Source: CAD feature listing. Evaluate the final solid. Frame: model axes, mm. Face numbers are marked on the shaded views. Round coordinates to 2 decimals unless told otherwise and drop trailing zeros. Write each loop counter-clockwise with the first axis right and the second up, starting at its lowest first coordinate (ties: lowest second). Pieces come first, ordered by that corner, then holes. Notation, with made-up numbers: (82, 28) -> (90, 28) arc R16 cw to (90, 39) -> close; hole circle Ø6 at (48, 84.25). An arc over 180 degrees is marked (long way). Put each result on its own line as item: value.
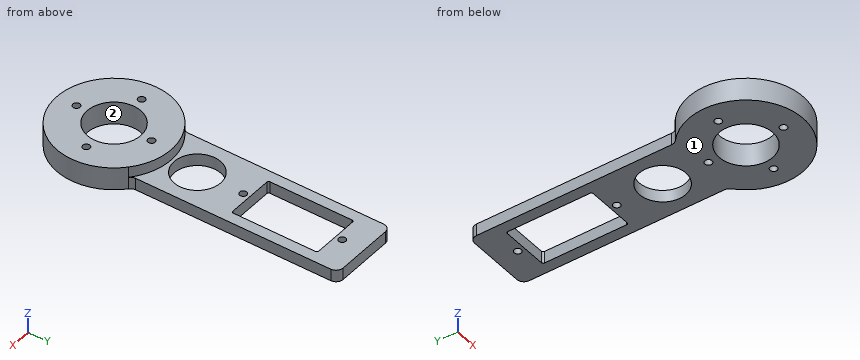
```python
from build123d import *
from build123d.topology import SkipClean

# Parameters (mm, degrees)
SKETCH1_R           = 1
BOSS_EXTRUDE1_DEPTH = 6.35
SKETCH2_R           = 1
SKETCH2_W           = 13.9
SKETCH2_H           = 24
CUT_EXTRUDE1_DEPTH  = 73.085522125
FILLET1_R           = 0.5
FILLET2_R           = 2
SKETCH3_R           = 6.5
CUT_EXTRUDE2_DEPTH  = 6.35
SKETCH4_R           = 7.5
CUT_EXTRUDE3_DEPTH  = 73.085522125
SKETCH5_R           = 6.5
SKETCH5_R_2         = 1
CUT_EXTRUDE4_DEPTH  = 3


with BuildPart() as part:
    # Sketch1 → Boss-Extrude1 (new body)
    with BuildSketch(Plane.XY):
        with BuildLine():
            Line((-10, 12.489995997), (-10, 70))
            Line((-10, 70), (10, 70))
            Line((10, 70), (10, 12.489995997))
            ThreePointArc((10, 12.489995997), (0, -16), (-10, 12.489995997))
        make_face()
        with Locations((-10.5, 0)):
            Circle(SKETCH1_R, mode=Mode.SUBTRACT)
        with Locations((0, 10.5)):
            Circle(SKETCH1_R, mode=Mode.SUBTRACT)
        with Locations((10.5, 0)):
            Circle(SKETCH1_R, mode=Mode.SUBTRACT)
        with Locations((0, -10.5)):
            Circle(SKETCH1_R, mode=Mode.SUBTRACT)
    extrude(amount=BOSS_EXTRUDE1_DEPTH)

    # Sketch2 → Cut-Extrude1 (cut, through all)
    with BuildSketch(Plane.XY.offset(6.35)):
        with Locations((0, 63.85)):
            Circle(SKETCH2_R)
        with Locations((0, 36.15)):
            Circle(SKETCH2_R)
        with Locations((0, 50)):
            Rectangle(SKETCH2_W, SKETCH2_H)
    extrude(amount=-CUT_EXTRUDE1_DEPTH, mode=Mode.SUBTRACT)

    # Fillet1
    fillet1_edges = [part.edges().sort_by_distance(p)[0] for p in [
        (6.95, 38, 3.175),
        (-6.95, 38, 3.175),
        (-6.95, 62, 3.175),
        (6.95, 62, 3.175),
    ]]
    fillet(fillet1_edges, radius=FILLET1_R)

    # Fillet2
    fillet2_edges = [part.edges().sort_by_distance(p)[0] for p in [
        (-10, 12.489995997, 3.175),
        (-10, 70, 3.175),
        (10, 70, 3.175),
        (10, 12.489995997, 3.175),
    ]]
    fillet(fillet2_edges, radius=FILLET2_R)

    # Sketch3 → Cut-Extrude2 (cut)
    with BuildSketch(Plane.XY.offset(6.35)):
        with Locations((0, 23.325)):
            Circle(SKETCH3_R)
    extrude(amount=-CUT_EXTRUDE2_DEPTH, mode=Mode.SUBTRACT)

    # Sketch4 → Cut-Extrude3 (cut, through all)
    with BuildSketch(Plane.XY.offset(6.35)):
        Circle(SKETCH4_R)
    extrude(amount=-CUT_EXTRUDE3_DEPTH, mode=Mode.SUBTRACT)

    # Sketch5 → Cut-Extrude4 (cut)
    with SkipClean():  # the faces are left unmerged after this step: merging them gives an invalid solid
        with BuildSketch(Plane.XY.offset(6.35)):
            with BuildLine():
                ThreePointArc((-10.666666667, 11.92569588), (0, 16), (10.666666667, 11.92569588))
                ThreePointArc((10.666666667, 11.92569588), (10.174258142, 12.599911284), (10, 13.416407865))
                Line((10, 13.416407865), (10, 68))
                ThreePointArc((10, 68), (9.414213562, 69.414213562), (8, 70))
                Line((8, 70), (-8, 70))
                ThreePointArc((-8, 70), (-9.414213562, 69.414213562), (-10, 68))
                Line((-10, 68), (-10, 13.416407865))
                ThreePointArc((-10, 13.416407865), (-10.174258142, 12.599911284), (-10.666666667, 11.92569588))
            make_face()
            with Locations((0, 23.325)):
                Circle(SKETCH5_R, mode=Mode.SUBTRACT)
            with Locations((0, 63.85)):
                Circle(SKETCH5_R_2, mode=Mode.SUBTRACT)
            with Locations((0, 36.15)):
                Circle(SKETCH5_R_2, mode=Mode.SUBTRACT)
            with BuildLine():
                ThreePointArc((6.45, 62), (6.803553391, 61.853553391), (6.95, 61.5))
                Line((6.95, 61.5), (6.95, 38.5))
                ThreePointArc((6.95, 38.5), (6.803553391, 38.146446609), (6.45, 38))
                Line((6.45, 38), (-6.45, 38))
                ThreePointArc((-6.45, 38), (-6.803553391, 38.146446609), (-6.95, 38.5))
                Line((-6.95, 38.5), (-6.95, 61.5))
                ThreePointArc((-6.95, 61.5), (-6.803553391, 61.853553391), (-6.45, 62))
                Line((-6.45, 62), (6.45, 62))
            make_face(mode=Mode.SUBTRACT)
        extrude(amount=-CUT_EXTRUDE4_DEPTH, mode=Mode.SUBTRACT)


solid = part.part
```
Q1. Cut plane A-A on x = 0. Give the number of separate pieces and of enclosed holes in the cut face, and give its area (3 significant figures).
Ans:
separate pieces: 8
enclosed holes: 0
area: 126 mm^2
Q2. Cut plane C-C on y = 0. Output: boundary loops of the cut face in (x, z), and give its area (4 significant figures).
Ans:
outline: (-16, 0) -> (-11.5, 0) -> (-11.5, 6.35) -> (-16, 6.35) -> close; (-9.5, 0) -> (-7.5, 0) -> (-7.5, 6.35) -> (-9.5, 6.35) -> close; (7.5, 0) -> (9.5, 0) -> (9.5, 6.35) -> (7.5, 6.35) -> close; (11.5, 0) -> (16, 0) -> (16, 6.35) -> (11.5, 6.35) -> close
area: 82.55 mm^2
Q3. Cut plane D-D on z = 5. Output: boundary loops of the cut face in (x, y), and give its area (3 significant figures).
Ans:
outline: circle Ø32 at (0, 0); hole circle Ø2 at (-10.5, 0); hole circle Ø15 at (0, 0); hole circle Ø2 at (0, -10.5); hole circle Ø2 at (0, 10.5); hole circle Ø2 at (10.5, 0)
area: 615 mm^2
Q4. Cut plane B-B on y = 36.15. Output: boundary loops of the cut face in (x, z).
Ans:
outline: (-10, 0) -> (-1, 0) -> (-1, 3.35) -> (-10, 3.35) -> close; (1, 0) -> (10, 0) -> (10, 3.35) -> (1, 3.35) -> close
Q5. Pin query (flat end, axial travel): pin 1 (1 mm diameter, centred on x = 7, y = 15.5, fed in from -Z); pin 2 (1.5 mm diameter, centred on x = 11.5, z = 3, fed in from +Y); pin 3 (6.5 mm diameter, centred on x = 0, y = 30, fed in from +Z); pin 4 (1.7 mm diameter, centred on y = 50.5, z = 2, fed in from -X). Return the tip coordinate at first contact, or that it passes through.
Ans:
pin 1: stops at z = 0
pin 2: stops at y = 11.85
pin 3: stops at z = 3.35
pin 4: stops at x = -10
Q6. Material intervals for line 1 (Y direction, x = -3, z = 3); line 2 (Y direction, x = 5.5, z = 3.25); line 3 (Y direction, x = 10.5, z = 4.5), sorted ascending. Write a range as [from, to].
Ans:
line 1: y = [-15.72, -6.87], [6.87, 17.56], [29.09, 38], [62, 70]
line 2: y = [-15.02, -5.1], [5.1, 19.86], [26.79, 38], [62, 70]
line 3: y = [-12.07, -1], [1, 12.07]
Q7. Draft query along Y for the marked faces 1 and 2. Return one class per face: +Y half, -Y half, draft (parallel to the pull), parting line (faces both ways), or undercut.
Ans:
face 1: draft
face 2: undercut
